Source: CAD feature listing. Evaluate the final solid. Frame: model axes, mm. A direction names the side the tool comes from. Coordinates: 2 decimals unless noted, no trailing zeros. Loops run counter-clockwise (first coordinate to the right, second up) from the corner with the lowest first, then second, coordinate; pieces in that order, holes last. Notation, with made-up numbers: M 17,74.25 L 37,74.25 A28 ccw 37,108.25 Z; hole C 33,31 d11. An arc over 180 degrees is marked long. One line per question, with ' | ' between items. Start each with the question number.
1. Ray query, probe 1 along Z at (x, y) = (20, -11) (3 decimals); probe 2 along Z at (x, y) = (-22, -14); probe 3 along X at (y, z) = (-8.5, -26.5). Return the intervals inside material, ascending.
2. Mould query, pull axis Y, two halves, no side actions, for faces 4 (the flat face through (25, -9, -29)), 5 (the flat face through (-0.8, -21.8, -19)), 6 (the flat face through (-18.368, -26.276, -16.435)), 7 (the cylindrical face through (0.318, -20.855, -15.294)). Classes: pulls with the +Y half, pulls with the -Y half, needs draft (parallel to the pull), parting line crosses it, or undercut.
3. Pin query (flat end, axial travel): P1, Ø1.5, axis at y = -6.5, z = -2, coming from the +X side; P2, Ø6, axis at x = -20, z = -25, coming from the +Y side (3 decimals); P3, Ø18, axis at x = -8, y = -24, coming from the -Z side; P4, Ø4.5, axis at x = 15, y = -6.6, coming from the +Z side. Return the tip coordinate at first contact, or that it passes through.
4. Access query for faces 1 (the cylindrical face through (0, -6, 35)), 2 (the flat face through (0, -21, -21)), 3 (the cylindrical face through (50.4, -8.67, 49.43)). Directions: +Z, -Z, +X, -X, +Y, -Y. A direction counts if a zero-diameter tool reaches every point of the face in a straight line with its end or side. Return the directions, or none.
5. Section query D-D, the plane x = 0. Output: boundary loops of the cut face in (y, z).
6. Section query A-A, the plane z = -25. Output: boundary loops of the cut face in (x, y) (3 decimals), and give its area (3 significant figures).
7. Section query C-C, the plane z = 45. Output: boundary loops of the cut face in (x, y) (3 decimals).
8. Section query B-B, the plane y = -10.5. Output: boundary loops of the cut face in (x, z) (3 decimals).
```python
from build123d import *

# Parameters (mm, degrees)
SKETCH025_R         = 2.325
PAD012_DEPTH        = 12
CHAMFER006_SIZE     = 5
FILLET_R            = 2
CHAMFER007_SIZE     = 0.7
SKETCH030_R         = 26
POCKET007_DEPTH     = 29.001
SKETCH031_R         = 10
PAD016_DEPTH        = 10
SKETCH032_R         = 11.15
POCKET008_DEPTH     = 8
CHAMFER008_SIZE     = 5
HOLE003_D           = 2.75
HOLE003_DEPTH       = 12
HOLE003_CSINK_D     = 3.8
HOLE003_CSINK_ANGLE = 90
HOLE003_TIPS_R      = 1.375
SKETCH034_W         = 51.071297
SKETCH034_H         = 46.191857
POCKET009_DEPTH     = 7.501
FILLET005_R         = 0.7
CHAMFER011_SIZE     = 0.69


with BuildPart() as part:
    # Sketch025 → Pad012 (new body)
    with BuildSketch(Plane.XZ):
        Polygon((-27, 50), (51, 50), (51, 40), (27, 16), (27, -32), (-27, -32), align=None)
        with Locations((-20, -25)):
            Circle(SKETCH025_R, mode=Mode.SUBTRACT)
        with Locations((-20, 45)):
            Circle(SKETCH025_R, mode=Mode.SUBTRACT)
        with Locations((20, 45)):
            Circle(SKETCH025_R, mode=Mode.SUBTRACT)
        with Locations((20, -25)):
            Circle(SKETCH025_R, mode=Mode.SUBTRACT)
    extrude(amount=PAD012_DEPTH)

    # Chamfer006
    chamfer006_edges = [part.edges().sort_by_distance(p)[0] for p in [
        (-27, -6, -32),
        (27, -6, -32),
    ]]
    chamfer(chamfer006_edges, length=CHAMFER006_SIZE)

    # Fillet
    fillet_edges = [part.edges().sort_by_distance(p)[0] for p in [
        (-22, -6, -32),
        (-27, -6, -27),
        (22, -6, -32),
        (27, -6, -27),
        (27, -6, 16),
        (51, -6, 40),
        (51, -6, 50),
        (-27, -6, 50),
    ]]
    fillet(fillet_edges, radius=FILLET_R)

    # Chamfer007
    chamfer007_edges = [part.edges().sort_by_distance(p)[0] for p in [
        (0, 0, -32),
        (21.93694, 0, -31.847759),
        (-21.93694, 0, -31.847759),
        (24.5, 0, -29.5),
        (-24.5, 0, -29.5),
        (26.847759, 0, -26.93694),
        (-26.847759, 0, -26.93694),
        (27, 0, -5.5),
        (-27, 0, 10.914214),
        (27.152241, 0, 15.93694),
        (-26.414214, 0, 49.414214),
        (39, 0, 28),
        (12, 0, 50),
        (50.847759, 0, 40.06306),
        (50.414214, 0, 49.414214),
        (51, 0, 44.414214),
        (17.675, 0, 45),
        (-22.325, 0, 45),
        (17.675, 0, -25),
        (-22.325, 0, -25),
        (0, -12, -32),
        (21.93694, -12, -31.847759),
        (-21.93694, -12, -31.847759),
        (24.5, -12, -29.5),
        (-24.5, -12, -29.5),
        (26.847759, -12, -26.93694),
        (-26.847759, -12, -26.93694),
        (27, -12, -5.5),
        (-27, -12, 10.914214),
        (27.152241, -12, 15.93694),
        (-26.414214, -12, 49.414214),
        (39, -12, 28),
        (12, -12, 50),
        (50.847759, -12, 40.06306),
        (50.414214, -12, 49.414214),
        (51, -12, 44.414214),
        (17.675, -12, 45),
        (-22.325, -12, 45),
        (17.675, -12, -25),
        (-22.325, -12, -25),
    ]]
    chamfer(chamfer007_edges, length=CHAMFER007_SIZE)

    # Sketch030 → Pocket007 (cut, through all)
    with BuildSketch(Plane(origin=(0, -29.4, 21), x_dir=(1, 0, 0), z_dir=(0, 0, 1))):
        Circle(SKETCH030_R)
    extrude(amount=POCKET007_DEPTH, mode=Mode.SUBTRACT)

    # Sketch031 → Pad016 (join)
    with BuildSketch(Plane(origin=(0, -29.4, -21), x_dir=(1, 0, 0), z_dir=(0, 0, 1))):
        with BuildLine():
            ThreePointArc((-11.905507, -6.36466), (0, -13.5), (11.905507, -6.36466))
            Line((26, 20), (11.905507, -6.36466))
            Line((-26, 20), (26, 20))
            Line((-11.905507, -6.36466), (-26, 20))
        make_face()
        Circle(SKETCH031_R, mode=Mode.SUBTRACT)
    extrude(amount=PAD016_DEPTH)

    # Sketch032 (on Face56 of Pad016) → Pocket008 (cut)
    with BuildSketch(Plane(origin=(0, 0, -11), x_dir=(-1, 0, 0), z_dir=(0, 0, 1))):
        with Locations((0, 29.4)):
            Circle(SKETCH032_R)
    extrude(amount=-POCKET008_DEPTH, mode=Mode.SUBTRACT)

    # Chamfer008
    chamfer008_edges = [part.edges().sort_by_distance(p)[0] for p in [
        (0, -12, -11),
    ]]
    chamfer(chamfer008_edges, length=CHAMFER008_SIZE)

    # Hole003
    with Locations(Plane(origin=(0, 0, 50), x_dir=(-1, 0, 0), z_dir=(0, 0, 1))):
        with Locations((15, 4), (-15, 4), (-27, 4), (-44, 4)):
            CounterSinkHole(HOLE003_D / 2, HOLE003_CSINK_D / 2, depth=HOLE003_DEPTH, counter_sink_angle=HOLE003_CSINK_ANGLE)

    # Hole003 tips → Hole003 tip 1 section 0
    with BuildSketch(Plane(origin=(0, 0, 38), x_dir=(-1, 0, 0), z_dir=(0, 0, 1)), mode=Mode.PRIVATE) as hole003_tip_1_s0:
        with Locations((15, 4)):
            Circle(HOLE003_TIPS_R)
    loft([hole003_tip_1_s0.sketch, Vertex(-15, -4, 37.173817)], mode=Mode.SUBTRACT)

    # Hole003 tips → Hole003 tip 2 section 0
    with BuildSketch(Plane(origin=(0, 0, 38), x_dir=(-1, 0, 0), z_dir=(0, 0, 1)), mode=Mode.PRIVATE) as hole003_tip_2_s0:
        with Locations((-15, 4)):
            Circle(HOLE003_TIPS_R)
    loft([hole003_tip_2_s0.sketch, Vertex(15, -4, 37.173817)], mode=Mode.SUBTRACT)

    # Hole003 tips → Hole003 tip 3 section 0
    with BuildSketch(Plane(origin=(0, 0, 38), x_dir=(-1, 0, 0), z_dir=(0, 0, 1)), mode=Mode.PRIVATE) as hole003_tip_3_s0:
        with Locations((-27, 4)):
            Circle(HOLE003_TIPS_R)
    loft([hole003_tip_3_s0.sketch, Vertex(27, -4, 37.173817)], mode=Mode.SUBTRACT)

    # Hole003 tips → Hole003 tip 4 section 0
    with BuildSketch(Plane(origin=(0, 0, 38), x_dir=(-1, 0, 0), z_dir=(0, 0, 1)), mode=Mode.PRIVATE) as hole003_tip_4_s0:
        with Locations((-44, 4)):
            Circle(HOLE003_TIPS_R)
    loft([hole003_tip_4_s0.sketch, Vertex(44, -4, 37.173817)], mode=Mode.SUBTRACT)

    # Sketch034 → Pocket009 (cut, through all)
    with BuildSketch(Plane.XZ.offset(35.4)):
        with Locations((1.865184, -14.980418)):
            Rectangle(SKETCH034_W, SKETCH034_H)
    extrude(amount=POCKET009_DEPTH, mode=Mode.SUBTRACT)

    # Fillet005
    fillet005_edges = [part.edges().sort_by_distance(p)[0] for p in [
        (-9.398005, -35.4, -15),
        (-8, -35.4, -20),
        (-12.100454, -35.4, -16),
        (9.398005, -35.4, -15),
        (12.100454, -35.4, -16),
        (8, -35.4, -20),
    ]]
    fillet(fillet005_edges, radius=FILLET005_R)

    # Chamfer011
    chamfer011_edges = [part.edges().sort_by_distance(p)[0] for p in [
        (17.11765, -26.01501, -11),
        (18.454145, -23.51501, -21),
    ]]
    chamfer(chamfer011_edges, length=CHAMFER011_SIZE)


with BuildPart() as part_1:
    # Body010 placement: moved
    add(part.part.moved(Location((0, -2.6, 0))))


solid = part_1.part
```
Taken from the geometry:
1) probe 1: -32 to -27.325, -22.675 to 42.675, 47.325 to 50 | probe 2: -31.71 to -26.37, -23.63 to 43.63, 46.37 to 49.9 | probe 3: -26.97 to -21.78, -18.22 to 18.22, 21.78 to 26.97
2) face 4: needs draft | face 5: undercut | face 6: pulls with the -Y half | face 7: undercut
3) P1: x = 27 | P2: y = -2.625 | P3: z = -21 | P4: z = 50
4) face 1: +Z, -Y | face 2: -Z, +X, -X, -Y | face 3: +Z, +X, +Y, -Y
5) outline: M -22,-20.31 L -21.31,-21 L -14.6,-21 L -14.6,-31.3 L -13.9,-32 L -3.3,-32 L -2.6,-31.3 L -2.6,49.3 L -3.3,50 L -6,50 L -6,21 L -14.6,21 L -14.6,-6 L -19.6,-11 L -20.16,-11 L -20.85,-11.69 L -20.85,-19 L -22,-19 Z
6) outline: M -27,-13.9 L -26.3,-14.6 L -23.025,-14.6 L -22.325,-13.9 L -22.325,-3.3 L -23.025,-2.6 L -26.3,-2.6 L -27,-3.3 Z; M -17.675,-13.9 L -16.975,-14.6 L 16.975,-14.6 L 17.675,-13.9 L 17.675,-3.3 L 16.975,-2.6 L -16.975,-2.6 L -17.675,-3.3 Z; M 22.325,-13.9 L 23.025,-14.6 L 26.3,-14.6 L 27,-13.9 L 27,-3.3 L 26.3,-2.6 L 23.025,-2.6 L 22.325,-3.3 Z | area: 533 mm^2
7) outline: M -27,-13.9 L -26.3,-14.6 L -23.025,-14.6 L -22.325,-13.9 L -22.325,-3.3 L -23.025,-2.6 L -26.3,-2.6 L -27,-3.3 Z; M -17.675,-12.932 A26 cw 17.675,-12.932 L 17.675,-3.3 L 16.975,-2.6 L -16.975,-2.6 L -17.675,-3.3 Z; M 22.325,-13.9 L 23.025,-14.6 L 50.3,-14.6 L 51,-13.9 L 51,-3.3 L 50.3,-2.6 L 23.025,-2.6 L 22.325,-3.3 Z; hole C -15,-6.6 d2.75; hole C 15,-6.6 d2.75; hole C 27,-6.6 d2.75; hole C 44,-6.6 d2.75
8) outline: M -27,-26.172 A2 ccw -26.414,-27.586 L -22.586,-31.414 A2 ccw -21.172,-32 L 21.172,-32 A2 ccw 22.586,-31.414 L 26.414,-27.586 A2 ccw 27,-26.172 L 27,15.172 A2 cw 27.586,16.586 L 50.414,39.414 A2 ccw 51,40.828 L 51,48 A2 ccw 49,50 L 14.62,50 L 14.62,21 L -14.62,21 L -14.62,50 L -25,50 A2 ccw -27,48 Z; hole C -20,-25 d4.65; hole C -20,45 d4.65; hole C 20,-25 d4.65; hole C 20,45 d4.65
